Build history of the part. All positions in model axes, mm. Coordinates: 2 decimals unless noted, no trailing zeros. Order: outer loops, then holes, each group sorted by start corner. A loop starts at its lowest first (then second) coordinate and runs counter-clockwise, first axis right, second up. Notation, with made-up numbers: M -29.75,-19.75 L 4.25,-19.75 A15 cw 4.25,-0.75 Z; hole C 14,-32 d8. An arc over 180 degrees is marked long. Use a Markdown table: item, result. Add a question column.
from build123d import *

# Parameters (mm, degrees)
BOSS_EXTRUDE1_DEPTH = 1


with BuildPart() as part:
    # Sketch1 → Boss-Extrude1 (new body)
    with BuildSketch(Plane.XY):
        with BuildLine():
            Line((208.284271247, -255), (255, -255))
            Line((255, -255), (255, 255))
            Line((255, 255), (-255, 255))
            Line((-255, 255), (-255, -255))
            Line((-255, -255), (-208.284271247, -255))
            ThreePointArc((-208.284271247, -255), (-202.510768556, -256.835034191), (-198.856180832, -261.666666667))
            ThreePointArc((-198.856180832, -261.666666667), (-180, -275), (-161.143819168, -261.666666667))
            ThreePointArc((-161.143819168, -261.666666667), (-157.489231444, -256.835034191), (-151.715728753, -255))
            Line((-151.715728753, -255), (151.715728753, -255))
            ThreePointArc((151.715728753, -255), (157.489231444, -256.835034191), (161.143819168, -261.666666667))
            ThreePointArc((161.143819168, -261.666666667), (180, -275), (198.856180832, -261.666666667))
            ThreePointArc((198.856180832, -261.666666667), (202.510768556, -256.835034191), (208.284271247, -255))
        make_face()
    extrude(amount=BOSS_EXTRUDE1_DEPTH)


solid = part.part
(1) Slice it at A-A on z = 0.25. Give the cut face in (x, y), and give its area (3 significant figures).
(2) Mould opens along X. For faces 1 (the flat face through (-4, -6, 0)), 2 (the cylindrical face through (179.655, -274.997, 0.493)) say: released by +X, released by -X, zero draft, split by the parting line, or undercut.
(3) Drill centre lines: line 1 along Y through (x, z) = (-30, 0.6); line 2 along Y through (x, z) = (153, 0.45). Where is each one in solid material? Low to high. Write a range as from..to.
(4) Slice it at B-B on x = -220. Give the cut face in (y, z).
Solutions:
| question | item | result |
|---|---|---|
| 1 | outline | M -255,-255 L -208.28,-255 A10 cw -198.86,-261.67 A20 ccw -161.14,-261.67 A10 cw -151.72,-255 L 151.72,-255 A10 cw 161.14,-261.67 A20 ccw 198.86,-261.67 A10 cw 208.28,-255 L 255,-255 L 255,255 L -255,255 Z |
| 1 | area | 261,000 mm² |
| 2 | face 1 | zero draft |
| 2 | face 2 | undercut |
| 3 | line 1 | -255..255 |
| 3 | line 2 | -255.08..255 |
| 4 | outline | M -255,0 L 255,0 L 255,1 L -255,1 Z |
